Could you check a few things on this model? Use its own coordinates, in mm. A direction names the side the tool comes from. Round coordinates to 2 decimals unless told otherwise and drop trailing zeros. Loops run counter-clockwise (first coordinate to the right, second up) from the corner with the lowest first, then second, coordinate; pieces in that order, holes last.
from build123d import *


with BuildPart() as part:
    # Sketch1 → Revolve-Thin1 (revolve)
    with BuildSketch(Plane.XY):
        with BuildLine():
            Line((0, 0), (3.175, 0))
            Line((3.175, 0), (3.175, 34.925))
            Line((3.175, 34.925), (5.5499, 34.925))
            ThreePointArc((5.5499, 34.925), (3.924371925, 38.849371925), (0, 40.4749))
            Line((0, 40.4749), (0, 37.9349))
            ThreePointArc((0, 37.9349), (0.840937575, 37.815038409), (1.614898762, 37.465))
            Line((1.614898762, 37.465), (0.635, 37.465))
            Line((0.635, 37.465), (0.635, 2.54))
            Line((0.635, 2.54), (0, 2.54))
            Line((0, 2.54), (0, 0))
        make_face()
    revolve(axis=Axis((0, 0, 0), (0, 1, 0)))


solid = part.part
Item 1: If we section it at B-B, the plane z = 0: Please give me the cut outline in (x, y) (3 decimals), then the cut area to 3 significant figures.
Results list:
outline: (-5.55, 34.925) - (-3.175, 34.925) - (-3.175, 0) - (3.175, 0) - (3.175, 34.925) - (5.55, 34.925) arc R5.55 ccw to start; hole (-1.615, 37.465) - (-0.635, 37.465) - (-0.635, 2.54) - (0.635, 2.54) - (0.635, 37.465) - (1.615, 37.465) arc R3.01 ccw to start
area: 225 mm2
Item 2: For faces 1 (the flat face through (-2.4, 34.925, 2.4)), 2 (the flat face through (1, 37.465, 0)), which set-ups out of +Z, -Z, +X, -X, +Y, -Y let a thin tool reach every point of the face, with its end or its side?
Results list:
face 1: -Y
face 2: none
Item 3: Will these pins go through, and if not, where does the flat tip stop? pin 1 (5 mm diameter, centred on x = 1.5, y = 12, fed in from -Z) (3 decimals); pin 2 (3 mm diameter, centred on x = 1.5, z = 2, fed in from +Y); pin 3 (1 mm diameter, centred on y = 25, z = -3, fed in from -X).
Results list:
pin 1: stops at z = -3.175
pin 2: stops at y = 40.38
pin 3: stops at x = -1.96
Item 4: If we section it at C-C, the plane y = 17: Please give me the cut outline in (x, z) (3 decimals), then the cut area to 3 significant figures.
Results list:
outline: circle Ø6.35 at (0, 0); hole circle Ø1.27 at (0, 0)
area: 30.4 mm2
Item 5: If we section it at D-D, the plane x = 2.25: Please give me the cut outline in (y, z) (3 decimals), then the cut area to 3 significant figures.
Results list:
outline: (0, -2.24) - (34.925, -2.24) - (34.925, -5.073) arc R5.073 ccw to (34.925, 5.073) - (34.925, 2.24) - (0, 2.24) - close
area: 197 mm2
Item 6: If we section it at A-A, the plane x = 0: Please give me the cut outline in (y, z) (3 decimals).
Results list:
outline: (0, -3.175) - (34.925, -3.175) - (34.925, -5.55) arc R5.55 ccw to (34.925, 5.55) - (34.925, 3.175) - (0, 3.175) - close; hole (2.54, -0.635) - (37.465, -0.635) - (37.465, -1.615) arc R3.01 ccw to (37.465, 1.615) - (37.465, 0.635) - (2.54, 0.635) - close
Item 7: If I drill on line 1 along Z through (x, y) = (0, 13) (3 decimals); line 2 along X through (y, z) = (4.5, 0.5), over which ranges is the centre line in solid material (lowest first)?
Results list:
line 1: z = -3.175 to -0.635, 0.635 to 3.175
line 2: x = -3.14 to -0.39, 0.39 to 3.14
Item 8: We'd pull the mould along Y, two halves only. Please class faces 3 (the cylindrical face through (-0.69, 17.71, 3.1)), 4 (the cylindrical face through (-0.08, 19.76, -0.63)), 5 (the flat face through (0, 0, 0)): released by +Y, released by -Y, zero draft, split by the parting line, or undercut.
Results list:
face 3: zero draft
face 4: undercut
face 5: released by -Y
